Autodesk Inventor part; units mm, degrees
ref_plane "YZ Plane" through (0, 0, 0) normal (1, 0, 0) x (0, 1, 0)
ref_plane "XZ Plane" through (0, 0, 0) normal (0, 1, 0) x (-1, 0, 0)
ref_plane "XY Plane" through (0, 0, 0) normal (0, 0, 1) x (1, 0, 0)
sketch "Sketch1" plane through (0, 0, 0) normal (0, 0, 1) x (1, 0, 0)
  line L0 (12.5729, -9.5) -> (10, -7.5)
  line L1 (10, -7.5) -> (-10, -7.5)
  line L2 (-10, -7.5) -> (-10, 7.5)
  line L3 (10, -7.5) -> (14.037, 12.0883)
  line L4 (14.037, 12.0883) -> (-10, 7.5)
  point P0 (0, 0)
  point P1 (-10, 0)
  dimension "d0" = 20
  dimension "d1" = 15
  dimension "d2" = 20
  dimension "d3" = 101.645
  dimension "d18" = 10
  dimension "d19" = 10
  dimension "d20" = 0
extrude "Extrusion1" add sketch "Sketch1" along normal blind 1
sketch "Sketch2" plane through (0, 0, 1) normal (0, 0, 1) x (1, 0, 0)
  line L0 (0.75, 5) -> (0.75, -5)
  line L1 (-0.75, -5) -> (-0.75, 5)
  line L2 (-0.75, 5) -> (-0.75, 6.5)
  line L3 (0.75, 6.5) -> (0.75, 5)
  line L4 (-0.75, -5) -> (-0.75, -7)
  line L5 (-0.75, -7) -> (0.75, -7)
  line L6 (0.75, -7) -> (0.75, -5)
  line L7 (-0.75, 6.5) -> (-0.75, 8.5)
  line L8 (-0.75, 8.5) -> (0.75, 8.5)
  line L9 (0.75, 8.5) -> (0.75, 6.5)
  point P0 (0, 0)
  point P1 (0.75, 0)
  dimension "d7" = 10
  dimension "d8" = 1.5
  dimension "d12" = 1.5
  dimension "d21" = 2
  dimension "d22" = 2
extrude "Extrusion2" add sketch "Sketch2" along normal blind 15
sketch "Sketch5" plane through (0.75, -7, 1) normal (1, 0, 0) x (0, 0, -1)
  line L0 (0, 15.5) -> (0, 0)
  line L1 (0, 15.5) -> (-15, 15.5)
  line L2 (-15, 0) -> (-15, 15.5)
  line L3 (0, 0) -> (-15, 0)
  line L4 (-15, 0) -> (-15, 1.5)
  line L5 (0, 15.5) -> (-1.5, 15.5)
  line L6 (-1.5, 15.5) -> (-15, 1.5)
  line L7 (-15, 1.5) -> (-15, 15.5)
  line L8 (-15, 15.5) -> (-1.5, 15.5)
  point P0 (1, 7)
  dimension "d23" = 1.5
  dimension "d24" = 1.5
extrude "Extrusion4" cut sketch "Sketch5" against normal through all contours L6 L2 L1
sketch "Sketch6" plane through (0.75, -7, 1) normal (1, 0, 0) x (0, 0, -1)
  circle A0 centre (-13.6955, 1.2065) radius 0.86
  circle A1 centre (-11.5498, 1.2065) radius 0.86
  circle A2 centre (-9.5052, 1.2065) radius 0.86
  circle A3 centre (-7.3796, 1.2065) radius 0.86
  circle A4 centre (-5.2541, 1.2065) radius 0.86
  circle A5 centre (-3.0678, 1.2065) radius 0.86
  point P0 (1, 7)
  dimension "d27" = 1.72
  dimension "d28" = 1.72
  dimension "d29" = 1.72
  dimension "d30" = 1.72
  dimension "d31" = 1.72
  dimension "d32" = 1.72
extrude "Extrusion5" cut sketch "Sketch6" against normal through all
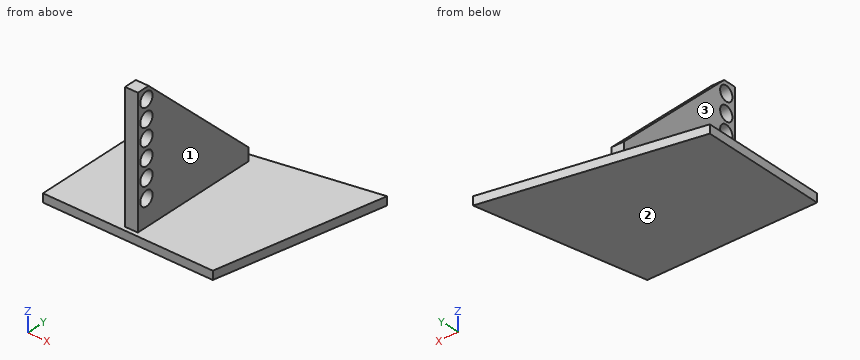
Model file for the job. Use its own axes, mm. Face numbers are marked on the shaded views. A direction names the side the tool comes from. Coordinates: 2 decimals unless noted, no trailing zeros. Write each loop counter-clockwise with the first axis right and the second up, starting at its lowest first coordinate (ties: lowest second). Pieces come first, ordered by that corner, then holes. Notation, with made-up numbers: (24, 50) - (64, 50) arc R28 ccw to (64, 73) - close; hole circle Ø7 at (24, 67.5). An arc over 180 degrees is marked (long way). Use a Markdown table: item, result. Add a question column.
Item 1: Drop flat-ended pins along their axis: pin 1 (1.5 mm diameter, centred on y = -5.79, z = 8.38, fed in from -X); pin 2 (3 mm diameter, centred on y = -5.79, z = 4.07, fed in from -X); pin 3 (2 mm diameter, centred on y = -5.79, z = 14.7, fed in from +X); pin 4 (6 mm diameter, centred on x = 1, y = 2.5, fed in from +Z). Give the stop position or say it passes through.
Item 2: Band-saw the part on A-A, the plane z = 4.5. Write the cut outline in (x, y), and give its area (3 significant figures).
Item 3: Band-saw the part on C-C, the plane z = 12. Write the cut outline in (x, y).
Item 4: Band-saw the part on D-D, the plane x = 2.5. Write the cut outline in (y, z), and give its area (3 significant figures).
Item 5: 3-axis set-ups, long thin cutter, end or side, ignore diameter. For the marked faces 1, 2 and 3: which of +Z, -Z, +X, -X, +Y, -Y reach the whole face in a straight line?
Item 6: Band-saw the part on B-B, the plane y = 2. Write the cut outline in (x, z).
Item 7: Drill centre lines: line 1 along X through (y, z) = (-1.25, 8.25); line 2 along Z through (x, y) = (-7.5, 3). Where is each one in solid material? Low to high.
A:
| question | item | result |
|---|---|---|
| 1 | pin 1 | passes through |
| 1 | pin 2 | stops at x = -0.75 |
| 1 | pin 3 | stops at x = 0.75 |
| 1 | pin 4 | stops at z = 11.17 |
| 2 | outline | (-0.75, -7) - (0.75, -7) - (0.75, -6.54) - (-0.75, -6.54) - close; (-0.75, -5.05) - (0.75, -5.05) - (0.75, 6.43) - (-0.75, 6.43) - close |
| 2 | area | 17.9 mm² |
| 3 | outline | (-0.75, -7) - (0.75, -7) - (0.75, -6.45) - (-0.75, -6.45) - close; (-0.75, -5.13) - (0.75, -5.13) - (0.75, -1.35) - (-0.75, -1.35) - close |
| 4 | outline | (-7.5, 0) - (9.89, 0) - (9.89, 1) - (-7.5, 1) - close |
| 4 | area | 17.4 mm² |
| 5 | face 1 | +Z, +X, +Y, -Y |
| 5 | face 2 | -Z, +X, -X, +Y, -Y |
| 5 | face 3 | +Z, -X, +Y, -Y |
| 6 | outline | (-10, 0) - (11.96, 0) - (11.96, 1) - (0.75, 1) - (0.75, 8.77) - (-0.75, 8.77) - (-0.75, 1) - (-10, 1) - close |
| 7 | line 1 | x = -0.75 to 0.75 |
| 7 | line 2 | z = 0 to 1 |
